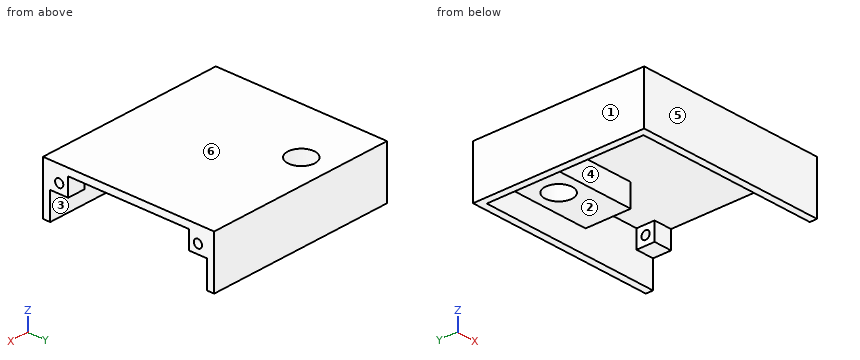
from build123d import *

# Parameters (mm, degrees)
SKETCH_1_W          = 210
SKETCH_1_H          = 190
EXTRUDE_1_DEPTH     = 8
EXTRUDE_2_DEPTH     = 50
SKETCH_3_W          = 20
SKETCH_3_H          = 20
EXTRUDE_3_DEPTH     = 20
SKETCH_8_R          = 4.55
CUT_EXTRUDE_1_DEPTH = 25
SKETCH_9_W          = 120
SKETCH_9_H          = 50
EXTRUDE_4_DEPTH     = 25
SKETCH_10_R         = 15
CUT_EXTRUDE_2_DEPTH = 146.392572025


with BuildPart() as part:
    # 스케치1 → 보스-돌출1 (new body)
    with BuildSketch(Plane.XY):
        Rectangle(SKETCH_1_W, SKETCH_1_H)
    extrude(amount=EXTRUDE_1_DEPTH)

    # 스케치2 → 보스-돌출2 (add)
    with BuildSketch(Plane(origin=(0, 0, 0), x_dir=(-1, 0, 0), z_dir=(0, 0, -1))):
        Polygon((-105, 95), (105, 95), (105, -95), (-105, -95), (-105, -87), (97, -87), (97, 87), (-105, 87), align=None)
    extrude(amount=EXTRUDE_2_DEPTH)

    # 스케치3 → 보스-돌출3 (add)
    with BuildSketch(Plane(origin=(105, 0, 0), x_dir=(0, 0, -1), z_dir=(1, 0, 0))):
        with Locations((10, 77)):
            Rectangle(SKETCH_3_W, SKETCH_3_H)
    extrude_3 = extrude(amount=-EXTRUDE_3_DEPTH)

    # 스케치8 → 컷-돌출1 (cut)
    with BuildSketch(Plane(origin=(105, 0, 0), x_dir=(0, 0, -1), z_dir=(1, 0, 0))):
        with Locations(Location((10, 77, 0), (0, 0, 90))):
            Circle(SKETCH_8_R)
    cut_extrude_1 = extrude(amount=-CUT_EXTRUDE_1_DEPTH, mode=Mode.SUBTRACT)

    # 대칭 복사1: 보스-돌출3, 컷-돌출1 across plane
    add(extrude_3.mirror(Plane(origin=(0, 0, 0), x_dir=(0, 0, 1), z_dir=(0, -1, 0))))
    add(cut_extrude_1.mirror(Plane(origin=(0, 0, 0), x_dir=(0, 0, 1), z_dir=(0, -1, 0))), mode=Mode.SUBTRACT)

    # 스케치9 → 보스-돌출4 (add)
    with BuildSketch(Plane(origin=(0, 0, 0), x_dir=(-1, 0, 0), z_dir=(0, 0, -1))):
        with Locations((37, 62)):
            Rectangle(SKETCH_9_W, SKETCH_9_H)
    extrude(amount=EXTRUDE_4_DEPTH)

    # 스케치10 → 컷-돌출2 (cut, through all)
    with BuildSketch(Plane(origin=(0, 0, -25), x_dir=(-1, 0, 0), z_dir=(0, 0, -1))):
        with Locations((37, 62)):
            Circle(SKETCH_10_R)
    extrude(amount=-CUT_EXTRUDE_2_DEPTH, mode=Mode.SUBTRACT)


solid = part.part
Input: part model. Units: mm. Frame: model coordinates. Face numbers are marked on the shaded views. A direction names the side the tool comes from. Coordinates: 2 decimals unless noted, no trailing zeros. Order: outer loops, then holes, each group sorted by start corner. A loop starts at its lowest first (then second) coordinate and runs counter-clockwise, first axis right, second up. Notation, with made-up numbers: M 15,60 L 67,60 A20 cw 67,86 Z; hole C 5,42.25 d8. An arc over 180 degrees is marked long. Answer as CSV lines item,"result".
1. Material intervals for line 1 (Y direction, x = -37, z = -5.5); line 2 (Y direction, x = 46.5, z = -1.5); line 3 (Z direction, x = 93.5, y = -77), sorted ascending. Write a range as from..to.
Reported:
line 1,"-95..-87, 37..47, 77..95"
line 2,"-95..-87, 87..95"
line 3,"-20..-14.55, -5.45..8"
2. Access query for the marked faces 1, 2 and 3. Directions: +Z, -Z, +X, -X, +Y, -Y. A direction counts if a zero-diameter tool reaches every point of the face in a straight line with its end or side. Return the directions, or none.
Reported:
face 1,"+Z, -Z, -X, +Y, -Y"
face 2,"-Z, +X"
face 3,"-Z"
3. First-contact query: P1, Ø6, axis at x = -69.5, y = -47, coming from the -Z side; P2, Ø6, axis at x = 92, y = -73.5, coming from the -Z side; P3, Ø1, axis at y = 54, z = -42, coming from the +X side; P4, Ø7.5, axis at y = 64.5, z = -15.5, coming from the +X side. Flat tips, straight axial feed; report the tip coordinate or a pass-through.
Reported:
P1,"z = 0"
P2,"z = -20"
P3,"x = -97"
P4,"x = 105"
4. Pull-direction query (Y, two-part tool) for the marked faces 4, 5 and 6; classes: released by +Y, released by -Y, zero draft, split by the parting line, or undercut.
Reported:
face 4,"undercut"
face 5,"released by -Y"
face 6,"zero draft"
5. Section C-C (x = -37). Return the cut outline in (y, z), then the cut area to 3 significant figures.
Reported:
outline,"M -95,-50 L -87,-50 L -87,0 L 37,0 L 37,-25 L 47,-25 L 47,8 L -95,8 Z; M 77,-25 L 87,-25 L 87,-50 L 95,-50 L 95,8 L 77,8 Z"
area,"2,580 mm2"
6. Section B-B (z = -10). Return the cut outline in (x, y).
Reported:
outline,"M -105,-95 L 105,-95 L 105,-81.55 L 85,-81.55 L 85,-87 L -97,-87 L -97,37 L 23,37 L 23,87 L 85,87 L 85,81.55 L 105,81.55 L 105,95 L -105,95 Z; M 85,-72.45 L 105,-72.45 L 105,-67 L 85,-67 Z; M 85,67 L 105,67 L 105,72.45 L 85,72.45 Z; hole C -37,62 d30"
7. Section A-A (y = -77). Return the cut outline in (x, z), then the cut area to 3 significant figures.
Reported:
outline,"M -105,-50 L -97,-50 L -97,0 L 85,0 L 85,-5.45 L 105,-5.45 L 105,8 L -105,8 Z; M 85,-20 L 105,-20 L 105,-14.55 L 85,-14.55 Z"
area,"2,300 mm2"
8. Section D-D (x = 56.5). Return the cut outline in (y, z), then the cut area to 3 significant figures.
Reported:
outline,"M -95,-50 L -87,-50 L -87,0 L 87,0 L 87,-50 L 95,-50 L 95,8 L -95,8 Z"
area,"2,320 mm2"
